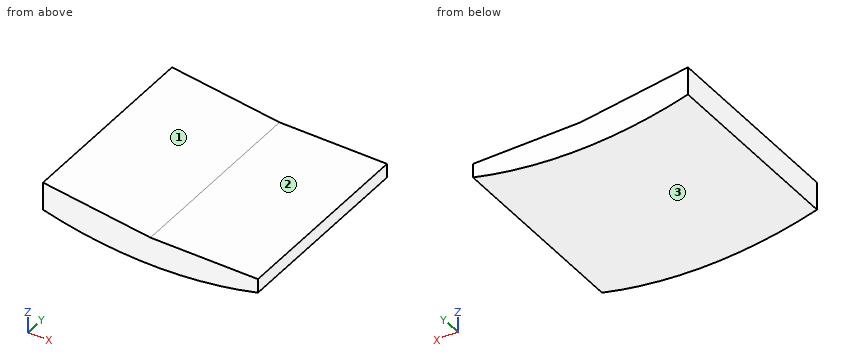
```python
from build123d import *

# Parameters (mm, degrees)
F1_DEPTH = 420


# Not quite as in the source:
# - a feature names something its author has since deleted; it is built from what else it names


with BuildPart() as f1:
    # F0 (on Front) → F1 (new body)
    with BuildSketch(Plane.XZ):
        Polygon((-230, -30), (0, -30), (-230, 0), align=None)
        Polygon((0, -30), (230, -30), (230, 0), (0, 0), (-230, 30), (-230, 0), align=None)
        with BuildLine():
            ThreePointArc((-230, -30), (0, -60), (230, -30))
            Line((230, -30), (0, -30))
            Line((0, -30), (-230, -30))
        make_face()
    extrude(amount=-F1_DEPTH)


solid = f1.part
```
Can you work these out from the model? Positions are in its coordinate system, mm. Face numbers are marked on the shaded views. Give positions to 0.01 mm unless a question says otherwise; leave off trailing zeros. Order: outer loops, then holes, each group sorted by start corner. A loop starts at its lowest first (then second) coordinate and runs counter-clockwise, first axis right, second up. Notation, with made-up numbers: (-5.75, 68.5) - (12.25, 68.5) arc R30 ccw to (12.25, 105.5) - close; hole circle Ø2 at (0, -14.5). An arc over 180 degrees is marked (long way). Use a Markdown table: item, result. Add a question column.
Q1. Please list where these lines run through material, in increasing order: line 1 along Z through (x, y) = (-196, 171.5); line 2 along Z through (x, y) = (163.5, 362.5).
Q2. If we section it at A-A on y = 137: Write out the boundary of the cut face in (x, z).
Q3. If we mould it in two halves opening along X, with no side actions, what happens to the marked faces 1, 2 and 3? For each: released by +X, released by -X, zero draft, split by the parting line, or undercut.
Q4. If we section it at B-B on z = 13.5: Write out the boundary of the cut face in (x, y), plus the area to 3 significant figures.
Q5. If we section it at C-C on x = 101: Write out the boundary of the cut face in (y, z).
Q6. I'm going to push flat-ended pins straight in: pin 1 (5 mm diameter, centred on x = 182, z = -42.5, fed in from -Y); pin 2 (1 mm diameter, centred on x = 91, y = 122.5, fed in from +Z). Where does each tip first touch, or does it pass through?
Answers follow:
| question | item | result |
|---|---|---|
| 1 | line 1 | z = -38.32 to 25.57 |
| 1 | line 2 | z = -44.97 to 0 |
| 2 | outline | (-230, -30) arc R896.67 ccw to (230, -30) - (230, 0) - (0, 0) - (-230, 30) - close |
| 3 | face 1 | released by +X |
| 3 | face 2 | zero draft |
| 3 | face 3 | split by the parting line |
| 4 | outline | (-230, 0) - (-103.5, 0) - (-103.5, 420) - (-230, 420) - close |
| 4 | area | 53,100 mm^2 |
| 5 | outline | (0, -54.29) - (420, -54.29) - (420, 0) - (0, 0) - close |
| 6 | pin 1 | stops at y = 0 |
| 6 | pin 2 | stops at z = 0 |
